Geometry check sheet. Reference: the model listing, model coordinates, mm. Face numbers are marked on the shaded views. Give positions to 0.01 mm unless a question says otherwise; leave off trailing zeros. Order: outer loops, then holes, each group sorted by start corner. A loop starts at its lowest first (then second) coordinate and runs counter-clockwise, first axis right, second up. Notation, with made-up numbers: M 43,89 L 57,89 A18 ccw 57,97 Z; hole C -6.75,85.5 d4. An arc over 180 degrees is marked long. Answer as CSV lines item,"result".
Autodesk Inventor part; units mm, degrees
ref_plane "YZ Plane" through (0, 0, 0) normal (1, 0, 0) x (0, 1, 0)
ref_plane "XZ Plane" through (0, 0, 0) normal (0, 1, 0) x (-1, 0, 0)
ref_plane "XY Plane" through (0, 0, 0) normal (0, 0, 1) x (1, 0, 0)
sketch "Sketch1" plane through (0, 0, 0) normal (0, 0, 1) x (1, 0, 0)
  line L0 (-21.0185, 21.59) -> (21.0185, 21.59)
  line L1 (21.0185, 21.59) -> (21.0185, -21.59)
  line L2 (21.0185, -21.59) -> (-21.0185, -21.59)
  line L3 (-21.0185, -21.59) -> (-21.0185, 21.59)
  point P0 (0, 0)
  dimension "d0" = 42.037
  dimension "d1" = 43.18
  dimension "d2" = 21.59
  dimension "d3" = 21.0185
extrude "Extrusion1" add sketch "Sketch1" along normal blind 42.672
sketch "Sketch2" plane through (0, 0, 42.672) normal (0, 0, 1) x (1, 0, 0)
  line L0 (21.0185, 21.59) -> (-21.0185, 21.59)
  line L1 (14.2875, 21.59) -> (14.2875, 14.859)
  line L2 (14.2875, 14.859) -> (21.0185, 14.859)
  line L3 (-21.0185, 21.59) -> (-21.0185, -21.59)
  line L4 (-21.0185, -14.859) -> (-14.2875, -14.859)
  line L5 (-14.2875, -14.859) -> (-14.2875, -21.59)
  line L6 (-21.0185, -21.59) -> (21.0185, -21.59)
  line L7 (21.0185, -21.59) -> (21.0185, 21.59)
  line L8 (14.2875, 21.59) -> (21.0185, 21.59)
  line L9 (21.0185, 21.59) -> (21.0185, 14.859)
  line L10 (-21.0185, -14.859) -> (-21.0185, -21.59)
  line L11 (-21.0185, -21.59) -> (-14.2875, -21.59)
  point P0 (0, 0)
  dimension "d6" = 6.731
  dimension "d7" = 6.731
  dimension "d8" = 6.731
  dimension "d9" = 6.731
  dimension "d10" = 0
extrude "Extrusion2" cut sketch "Sketch2" against normal blind 25.4 contours L7 L2 L1 L0 | L4 L5 L6 L3
equation "\"d6\" = d7"
equation "\"d8\" = d7"
equation "\"d9\" = d8"
properties part number "Transmission"
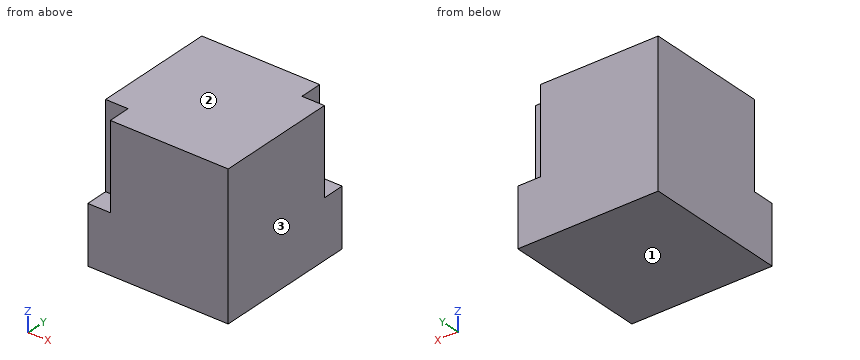
(1) Section check A-A on x = -15.5. Enter the section's corners in (y, z).
The answers:
outline,"M -21.59,0 L 21.59,0 L 21.59,42.67 L -14.86,42.67 L -14.86,17.27 L -21.59,17.27 Z"
(2) Gauge pin test, flat ends, axial feed: P1, Ø2, axis at x = -8.5, y = -2.5, coming from the -Z side; P2, Ø7.5, axis at x = -18.5, z = 27, coming from the -Y side. Record the tip position at first contact, or that the pin passes through.
The answers:
P1,"stops at z = 0"
P2,"stops at y = -14.86"
(3) Draft check along Z on the marked faces 1, 2 and 3. Enter one of: +Z half, -Z half, draft (parallel to the pull), parting line (faces both ways), or undercut.
The answers:
face 1,"-Z half"
face 2,"+Z half"
face 3,"draft"
(4) Section check C-C on y = -18. Enter the section's corners in (x, z), then the cut area to 3 significant figures.
The answers:
outline,"M -21.02,0 L 21.02,0 L 21.02,42.67 L -14.29,42.67 L -14.29,17.27 L -21.02,17.27 Z"
area,"1,620 mm2"
(5) Section check B-B on z = 20.5. Enter the section's corners in (x, y), then the cut area to 3 significant figures.
The answers:
outline,"M -21.02,-14.86 L -14.29,-14.86 L -14.29,-21.59 L 21.02,-21.59 L 21.02,14.86 L 14.29,14.86 L 14.29,21.59 L -21.02,21.59 Z"
area,"1,720 mm2"
(6) Material ranges on line 1 (Y direction, x = 17, z = 34); line 2 (X direction, y = -17, z = 27); line 3 (X direction, y = 15.5, z = 31), recorded low to high.
The answers:
line 1,"y = -21.59 to 14.86"
line 2,"x = -14.29 to 21.02"
line 3,"x = -21.02 to 14.29"
